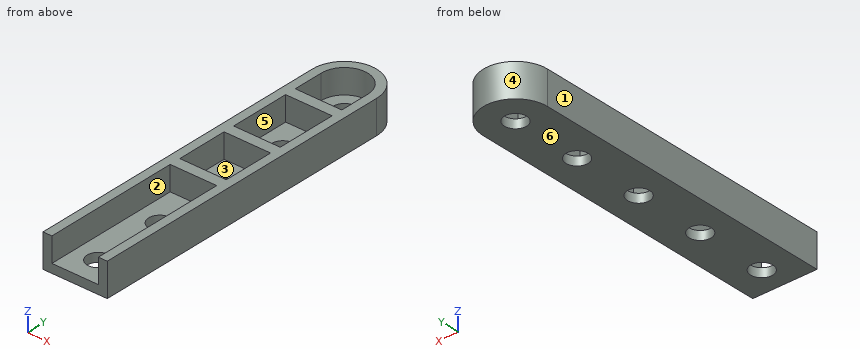
from build123d import *

# Parameters (mm, degrees)
F1_DEPTH = 9.525
F2_T     = -2.54
F3_W     = 13.335
F3_H     = 2.54
F4_DEPTH = 6.985
F5_R     = 3.175
F6_DEPTH = 2.541
F7_W     = 13.335
F7_H     = 3.175
F8_DEPTH = 6.985


with BuildPart() as f1:
    # F0 (on Top) → F1 (new body)
    with BuildSketch(Plane.XY):
        with BuildLine():
            Line((-9.2075, 88.9), (-9.2075, 0))
            Line((-9.2075, 0), (9.2075, 0))
            Line((9.2075, 0), (9.2075, 88.9))
            ThreePointArc((9.2075, 88.9), (0, 98.1075), (-9.2075, 88.9))
        make_face()
    extrude(amount=F1_DEPTH)

    # F2
    f2_openings = [f1.faces().sort_by_distance(p)[0] for p in [
        (0, 48.087743, 9.525),
    ]]
    offset(amount=F2_T, openings=f2_openings)

    # F3 (on face) → F4 (cut, through all)
    with BuildSketch(Plane.XY.offset(9.525)):
        with Locations((0, 1.27)):
            Rectangle(F3_W, F3_H)
    extrude(amount=-F4_DEPTH, mode=Mode.SUBTRACT)

    # F5 (on face) → F6 (cut, through all)
    with BuildSketch(Plane.XY.offset(2.54)):
        with Locations((0, 88.9)):
            Circle(F5_R)
        with Locations((0, 68.58)):
            Circle(F5_R)
        with Locations((0, 48.26)):
            Circle(F5_R)
        with Locations((0, 27.94)):
            Circle(F5_R)
        with Locations((0, 7.62)):
            Circle(F5_R)
    extrude(amount=-F6_DEPTH, mode=Mode.SUBTRACT)

    # F7 (on face) → F8 (join, through all)
    with BuildSketch(Plane.XY.offset(2.54)):
        with Locations((0, 78.74)):
            Rectangle(F7_W, F7_H)
        with Locations((0, 58.42)):
            Rectangle(F7_W, F7_H)
        with Locations((0, 40.64)):
            Rectangle(F7_W, F7_H)
    extrude(amount=F8_DEPTH)


solid = f1.part
Part model, mm, in its own coordinate system. Face numbers are marked on the shaded views. A direction names the side the tool comes from. Coordinates: 2 decimals unless noted, no trailing zeros. Loops run counter-clockwise (first coordinate to the right, second up) from the corner with the lowest first, then second, coordinate; pieces in that order, holes last. Notation, with made-up numbers: (58, 25) -> (65, 25) arc R34 cw to (65, 58) -> close; hole circle Ø6 at (41, 51). An arc over 180 degrees is marked (long way). Use a Markdown table: item, result. Add a question column.
Item 1: Band-saw the part on B-B on z = 3.5. Write the cut outline in (x, y) (1 decimal).
Item 2: Pull direction Y, two halves, no side cores. Call the marked faces 4, 5 and 6: +Y half, -Y half, draft (parallel to the pull), parting line (faces both ways), or undercut.
Item 3: Probe probe 1 along Y at (x, z) = (0, 1.8) (1 decimal); probe 2 along X at (y, z) = (68.5, 4.5); probe 3 along Y at (x, z) = (3.5, 5) (1 decimal). List the from-to ranges inside material, lowest first.
Item 4: Flat gauge pins, fed straight in: P1, Ø5.5, axis at x = 0, y = 27.94, coming from the -Z side; P2, Ø6.5, axis at x = 0, y = 14, coming from the +Z side; P3, Ø2, axis at x = 1, z = 7.5, coming from the -Y side. Where does each tip first touch, or does it go through?
Item 5: Band-saw the part on A-A on y = 7.62. Write the cut outline in (x, z) (1 decimal).
Item 6: Band-saw the part on C-C on x = 0. Give the number of separate pieces and of enclosed holes in the cut face, plus the area to 3 significant figures.
Item 7: Which spindle directions (+Z, -Z, +X, -X, +Y, -Y) get a long thin tool onto all of the face, cutting with end or side? Do the marked faces 1, 2 and 3. Say none if no direction does.
Item 8: Band-saw the part on D-D on y = 19. Write the cut outline in (x, z) (1 decimal).
Geometry says:
| question | item | result |
|---|---|---|
| 1 | outline | (-9.2, 0) -> (-6.7, 0) -> (-6.7, 39.1) -> (6.7, 39.1) -> (6.7, 0) -> (9.2, 0) -> (9.2, 88.9) arc R9.2 ccw to (-9.2, 88.9) -> close; hole (-6.7, 42.2) -> (6.7, 42.2) -> (6.7, 56.8) -> (-6.7, 56.8) -> close; hole (-6.7, 60) -> (6.7, 60) -> (6.7, 77.2) -> (-6.7, 77.2) -> close; hole (-6.7, 80.3) -> (6.7, 80.3) -> (6.7, 88.9) arc R6.7 ccw to (-6.7, 88.9) -> close |
| 2 | face 4 | +Y half |
| 2 | face 5 | undercut |
| 2 | face 6 | draft |
| 3 | probe 1 | 0 to 4.4, 10.8 to 24.8, 31.1 to 45.1, 51.4 to 65.4, 71.8 to 85.7, 92.1 to 98.1 |
| 3 | probe 2 | -9.21 to -6.67, 6.67 to 9.21 |
| 3 | probe 3 | 39.1 to 42.2, 56.8 to 60, 77.2 to 80.3, 94.6 to 97.4 |
| 4 | P1 | through |
| 4 | P2 | z = 2.54 |
| 4 | P3 | y = 39.05 |
| 5 | outline | (-9.2, 0) -> (-3.2, 0) -> (-3.2, 2.5) -> (-6.7, 2.5) -> (-6.7, 9.5) -> (-9.2, 9.5) -> close; (3.2, 0) -> (9.2, 0) -> (9.2, 9.5) -> (6.7, 9.5) -> (6.7, 2.5) -> (3.2, 2.5) -> close |
| 6 | separate pieces | 6 |
| 6 | enclosed holes | 0 |
| 6 | area | 253 mm² |
| 7 | face 1 | +Z, -Z, -X, +Y, -Y |
| 7 | face 2 | +Z, -Y |
| 7 | face 3 | +Z |
| 8 | outline | (-9.2, 0) -> (9.2, 0) -> (9.2, 9.5) -> (6.7, 9.5) -> (6.7, 2.5) -> (-6.7, 2.5) -> (-6.7, 9.5) -> (-9.2, 9.5) -> close |
